from build123d import *

# Parameters (mm, degrees)
SKETCH2_W           = 50
SKETCH2_H           = 100
BOSS_EXTRUDE1_DEPTH = 25
SKETCH5_W           = 30
SKETCH5_H           = 25
BOSS_EXTRUDE3_DEPTH = 8
SKETCH6_R           = 5
BOSS_EXTRUDE4_DEPTH = 30


with BuildPart() as part:
    # Sketch2 → Boss-Extrude1 (new body)
    with BuildSketch(Plane.XY):
        Rectangle(SKETCH2_W, SKETCH2_H)
    extrude(amount=-BOSS_EXTRUDE1_DEPTH)

    # Sketch5 → Boss-Extrude3 (add)
    with BuildSketch(Plane.XY):
        with Locations((0, 30)):
            Rectangle(SKETCH5_W, SKETCH5_H)
    extrude(amount=BOSS_EXTRUDE3_DEPTH)

    # Sketch6 → Boss-Extrude4 (add)
    with BuildSketch(Plane.XY.offset(8)):
        with Locations((0, 30)):
            Circle(SKETCH6_R)
    extrude(amount=BOSS_EXTRUDE4_DEPTH)


solid = part.part
Read the model definition and answer for the solid it produces. Units are mm, in the model's axes. A direction names the side the tool comes from. Round coordinates to 2 decimals unless told otherwise and drop trailing zeros. Order: outer loops, then holes, each group sorted by start corner. A loop starts at its lowest first (then second) coordinate and runs counter-clockwise, first axis right, second up.
1) The part is cut by section D-D on y = 19. Write down the section's boundary in (x, z), plus the area to 3 significant figures.
2) The part is cut by section C-C on z = 19.5. Write down the section's boundary in (x, y).
3) For faces 1 (the face through (0, 42.5, 4)), 2 (the face through (-15, 30, 4)), 3 (the face through (0, 17.5, 4)), 4 (the face through (-1.08, 25.12, 22.79)), determine the directions among +Z, -Z, +X, -X, +Y, -Y from which every point of the face is accessible in a straight line to the end or side of a thin tool.
4) Flat-ended cylindrical pins translate along their axes: pin 1 (10 mm diameter, centred on x = 11, y = -37, fed in from +Z); pin 2 (4 mm diameter, centred on x = -3.5, z = 5, fed in from +Y); pin 3 (6.5 mm diameter, centred on x = 4, z = 5.5, fed in from -Y). Find the tip coordinate at first contact, or state that the pin passes through.
5) The part is cut by section B-B on y = 30. Write down the section's boundary in (x, z).
6) The part is cut by section A-A on x = 0. Write down the section's boundary in (y, z), plus the area to 3 significant figures.
7) Straight lines are drawn through the part: L1, parallel to Z at x = -1, y = 21; L2, parallel to Z at x = -22, y = 1.5; L3, parallel to Y at x = 2, z = 20. For each, find the intervals that lie inside material, in ascending order.
Resolved:
1. outline: (-25, -25) - (25, -25) - (25, 0) - (15, 0) - (15, 8) - (-15, 8) - (-15, 0) - (-25, 0) - close
1. area: 1,490 mm2
2. outline: circle Ø10 at (0, 30)
3. face 1: +Z, +X, -X, +Y
3. face 2: +Z, -X, +Y, -Y
3. face 3: +Z, +X, -X, -Y
3. face 4: +Z
4. pin 1: stops at z = 0
4. pin 2: stops at y = 42.5
4. pin 3: stops at y = 17.5
5. outline: (-25, -25) - (25, -25) - (25, 0) - (15, 0) - (15, 8) - (5, 8) - (5, 38) - (-5, 38) - (-5, 8) - (-15, 8) - (-15, 0) - (-25, 0) - close
6. outline: (-50, -25) - (50, -25) - (50, 0) - (42.5, 0) - (42.5, 8) - (35, 8) - (35, 38) - (25, 38) - (25, 8) - (17.5, 8) - (17.5, 0) - (-50, 0) - close
6. area: 3,000 mm2
7. L1: z = -25 to 8
7. L2: z = -25 to 0
7. L3: y = 25.42 to 34.58
